```python
from build123d import *
from OCP.BRepFilletAPI import BRepFilletAPI_MakeChamfer

# Parameters (mm, degrees)
SKETCH_1_W               = 87
SKETCH_1_H               = 48
EXTRUDE_1_DEPTH          = 12
SKETCH_3_W               = 75
SKETCH_3_H               = 30
CUT_EXTRUDE_1_DEPTH      = 3
SKETCH_4_R               = 6
CUT_EXTRUDE_2_DEPTH      = 52.110175112
SKETCH_5_W               = 87
SKETCH_5_H               = 9
EXTRUDE_2_DEPTH          = 21
SKETCH_7_R               = 19.5
EXTRUDE_3_DEPTH          = 24
SKETCH_8_R               = 9
CUT_EXTRUDE_3_DEPTH      = 17
EXTRUDE_4_DEPTH          = 4.5
CUT_EXTRUDE_4_REACH      = 98.444
CUT_EXTRUDE_4_END_RADIUS = 9
SKETCH_13_R              = 3
CHAMFER_6_SIZE           = 1
CHAMFER_6_SIZE2          = 0.14060595
CHAMFER_6_SIZE2_2        = 0.017455065


with BuildPart() as part:
    # Sketch 1 → Extrude 1 (new body)
    with BuildSketch(Plane.XY):
        Rectangle(SKETCH_1_W, SKETCH_1_H)
    extrude(amount=-EXTRUDE_1_DEPTH)

    # Sketch 3 → Cut-Extrude 1 (cut)
    with BuildSketch(Plane(origin=(0, 0, -12), x_dir=(-1, 0, 0), z_dir=(0, 0, -1))):
        Rectangle(SKETCH_3_W, SKETCH_3_H)
    extrude(amount=-CUT_EXTRUDE_1_DEPTH, mode=Mode.SUBTRACT)

    # Sketch 4 → Cut-Extrude 2 (cut, through all)
    with BuildSketch(Plane.XY):
        with Locations((24, 0)):
            Circle(SKETCH_4_R)
        with Locations((-24, 0)):
            Circle(SKETCH_4_R)
    extrude(amount=-CUT_EXTRUDE_2_DEPTH, mode=Mode.SUBTRACT)

    # Sketch 5 → Extrude 2 (add)
    with BuildSketch(Plane(origin=(0, 0, -12), x_dir=(-1, 0, 0), z_dir=(0, 0, -1))):
        with Locations((0, -19.5)):
            Rectangle(SKETCH_5_W, SKETCH_5_H)
    extrude(amount=EXTRUDE_2_DEPTH)



with BuildPart() as body_2:
    # Sketch 7 → Extrude 3 (new, symmetric)
    with BuildSketch(Plane.XY.offset(-6)):
        with Locations((0, -75)):
            Circle(SKETCH_7_R)
    extrude(amount=EXTRUDE_3_DEPTH, both=True)

    # Sketch 8 → Cut-Extrude 3 (cut, symmetric)
    with BuildSketch(Plane.XY.offset(-6)):
        with Locations((0, -75)):
            Circle(SKETCH_8_R)
    extrude(amount=CUT_EXTRUDE_3_DEPTH, both=True, mode=Mode.SUBTRACT)

    # Sketch 10 → Cut-Revolve 1 (revolve, cut)
    with BuildSketch(Plane(origin=(0, -75, 0), x_dir=(1, 0, 0), z_dir=(0, 1, 0))):
        Polygon((0, -18), (0, -11), (9, -11), (10, -18), align=None)
    cut_revolve_1 = revolve(axis=Axis((0, -75, 18), (0, 0, -1)), mode=Mode.SUBTRACT)

    # Mirror 1: Cut-Revolve 1 across plane
    add(cut_revolve_1.mirror(Plane.XY.offset(-6)), mode=Mode.SUBTRACT)


with BuildPart() as part_1:
    add(part.part)

    add(body_2.part)  # Extrude 4 merges body 2
    # Sketch 12 → Extrude 4 (add, symmetric)
    with BuildSketch(Plane.XY.offset(-6)):
        with BuildLine():
            Line((-29.942238006, -27.63856044), (-15.687432014, -60.934386997))
            ThreePointArc((-15.687432014, -60.934386997), (-15.461093284, -62.422417649), (-15.985936875, -63.83309254))
            ThreePointArc((-15.985936875, -63.83309254), (0, -55.5), (15.985936875, -63.83309254))
            ThreePointArc((15.985936875, -63.83309254), (15.461093284, -62.422417649), (15.687432014, -60.934386997))
            Line((15.687432014, -60.934386997), (29.942238006, -27.63856044))
            ThreePointArc((29.942238006, -27.63856044), (32.154108719, -24.99157523), (35.457997537, -24))
            Line((35.457997537, -24), (-35.457997537, -24))
            ThreePointArc((-35.457997537, -24), (-32.154108719, -24.99157523), (-29.942238006, -27.63856044))
        make_face()
    extrude(amount=EXTRUDE_4_DEPTH, both=True)

    # Cut-Extrude 4: up to this cylinder (the profile starts outside it)
    cut_extrude_4_end = Plane(origin=(0, -75, 6), z_dir=(0, 0, 1)) * Cylinder(CUT_EXTRUDE_4_END_RADIUS, 215.888, mode=Mode.PRIVATE)
    # Sketch 13 → Cut-Extrude 4 (cut, up to the surface)
    with BuildSketch(Plane(origin=(0, -55.5, 0), x_dir=(1, 0, 0), z_dir=(0, 1, 0)), mode=Mode.PRIVATE) as cut_extrude_4_sk1:
        with Locations(Location((0, -6, 0), (0, 0, 270))):
            Circle(SKETCH_13_R)
    cut_extrude_4_tool1 = extrude(cut_extrude_4_sk1.sketch, amount=-CUT_EXTRUDE_4_REACH, mode=Mode.PRIVATE) - cut_extrude_4_end
    add(cut_extrude_4_tool1.solids().sort_by_distance((0, -55.5, 6))[0], mode=Mode.SUBTRACT)

    # Sketch 14 → Cut-Revolve 2 (revolve, cut)
    with BuildSketch(Plane.XY.offset(6), mode=Mode.PRIVATE) as cut_revolve_2_sk:
        Polygon((0, -55.5), (0, -57.5), (3, -57.5), (4.5, -55.5), align=None)
    revolve(cut_revolve_2_sk.sketch.rotate(Axis((0, -55.5, 6), (0, -1, 0)), 90), axis=Axis((0, -55.5, 6), (0, -1, 0)), mode=Mode.SUBTRACT)

    # Chamfer 6: one chamfer whose edges measure the first distance from different faces: ONE call of the kernel's chamfer builder (chamfer() names one face for all edges)
    chamfer_6_edges_1 = [part_1.edges().sort_by_distance(p)[0] for p in [
        (-9, -75, 11),
    ]]
    chamfer_6_side_1 = [part_1.faces().sort_by_distance(p)[0] for p in [
        (-9.5, -75, 14.5),
    ]]
    chamfer_6_edges_2 = [part_1.edges().sort_by_distance(p)[0] for p in [
        (-19.5, -75, -30),
    ]]
    chamfer_6_side_2 = [part_1.faces().sort_by_distance(p)[0] for p in [
        (-18.948456711, -75, -30),
    ]]
    chamfer_6_edges_3 = [part_1.edges().sort_by_distance(p)[0] for p in [
        (-19.5, -75, 18),
    ]]
    chamfer_6_side_3 = [part_1.faces().sort_by_distance(p)[0] for p in [
        (-19.5, -75, -6),
    ]]
    chamfer_6_edges_4 = [part_1.edges().sort_by_distance(p)[0] for p in [
        (-9, -75, -23),
    ]]
    chamfer_6_side_4 = [part_1.faces().sort_by_distance(p)[0] for p in [
        (-9, -75, -6),
    ]]
    chamfer_6 = BRepFilletAPI_MakeChamfer(part_1.part.solid().wrapped)
    for e in chamfer_6_edges_1:
        chamfer_6.Add(CHAMFER_6_SIZE, CHAMFER_6_SIZE2, e.wrapped, chamfer_6_side_1[0].wrapped)  # the first distance lies on this face
    for e in chamfer_6_edges_2:
        chamfer_6.Add(CHAMFER_6_SIZE, CHAMFER_6_SIZE2_2, e.wrapped, chamfer_6_side_2[0].wrapped)  # the first distance lies on this face
    for e in chamfer_6_edges_3:
        chamfer_6.Add(CHAMFER_6_SIZE, CHAMFER_6_SIZE2_2, e.wrapped, chamfer_6_side_3[0].wrapped)  # the first distance lies on this face
    for e in chamfer_6_edges_4:
        chamfer_6.Add(CHAMFER_6_SIZE, CHAMFER_6_SIZE2, e.wrapped, chamfer_6_side_4[0].wrapped)  # the first distance lies on this face
    add(Compound.cast(chamfer_6.Shape()), mode=Mode.REPLACE)


solid = part_1.part
```
Can you work these out from the model? Positions are in its coordinate system, mm. A direction names the side the tool comes from. Coordinates: 2 decimals unless noted, no trailing zeros. Loops run counter-clockwise (first coordinate to the right, second up) from the corner with the lowest first, then second, coordinate; pieces in that order, holes last.
Item 1: Suppose I cut it at C-C (x = -24). Please give me the cut outline in (y, z).
Answers below:
outline: (-41.52, -10.5) - (-24, -10.5) - (-24, -33) - (-15, -33) - (-15, -9) - (-6, -9) - (-6, 0) - (-24, 0) - (-24, -1.5) - (-41.52, -1.5) - close; (6, -9) - (15, -9) - (15, -12) - (24, -12) - (24, 0) - (6, 0) - close
Item 2: Which directions (+Z, -Z, +X, -X, +Y, -Y) give clear straight access to the entire face, cutting with the end or side of a thin tool? Please do faces 5 (the face through (37.5, 0, -11)), 6 (the face through (-1, 18, -12)), 7 (the face through (-4.227, -94.036, -6.162)), 8 (the face through (-1, 0, 0)).
Answers below:
face 5: -Z
face 6: -Z, +X, -X, +Y
face 7: none
face 8: +Z, +X, -X, +Y
Item 3: If we mould it in two halves opening along Y, with no side actions, what happens to faces 1 (the face through (-1.15, -61.94, 8.77)), 2 (the face through (1, 15, -11)), 3 (the face through (0, -39, -1.5)), 4 (the face through (-1, 24, -6))? For each: released by +Y, released by -Y, zero draft, split by the parting line, or undercut.
Answers below:
face 1: zero draft
face 2: undercut
face 3: undercut
face 4: released by +Y
Item 4: I'm going to push flat-ended pins straight in: pin 1 (3 mm diameter, centred on y = -79.5, z = -20.5, fed in from +X); pin 2 (12 mm diameter, centred on x = -1.5, y = -36, fed in from +Z); pin 3 (12 mm diameter, centred on y = -71, z = -9, fed in from +X); pin 4 (12 mm diameter, centred on y = 7, z = 3.5, fed in from +X). Where does each tip first touch, or does it pass through?
Answers below:
pin 1: stops at x = 19.27
pin 2: stops at z = -1.5
pin 3: stops at x = 19.5
pin 4: stops at x = 43.5
Item 5: Please list where these lines run through material, in increasing order: L1, parallel to Z at x = 0, y = -60.5; L2, parallel to Y at x = -5.5, z = -15; L3, parallel to Y at x = 20.5, z = -27.5.
Answers below:
L1: z = -30 to 3, 9 to 18
L2: y = -93.71 to -82.12, -67.88 to -56.29, -24 to -15
L3: y = -24 to -15
Item 6: Suppose I cut it at B-B (x = 26.5). Please give me the cut outline in (y, z).
Answers below:
outline: (-35.68, -10.5) - (-24, -10.5) - (-24, -33) - (-15, -33) - (-15, -9) - (-5.45, -9) - (-5.45, 0) - (-24, 0) - (-24, -1.5) - (-35.68, -1.5) - close; (5.45, -9) - (15, -9) - (15, -12) - (24, -12) - (24, 0) - (5.45, 0) - close
Item 7: Suppose I cut it at D-D (z = 6). Please give me the cut outline in (x, y), then the cut area to 4 significant figures.
Answers below:
outline: (-4.16, -55.95) arc R19.5 ccw (long way) to (4.16, -55.95) - (3, -57.5) - (3, -66.51) arc R9 cw (long way) to (-3, -66.51) - (-3, -57.5) - close
area: 874.5 mm2
Item 8: Suppose I cut it at A-A (y = 0). Please give me the cut outline in (x, z).
Answers below:
outline: (-43.5, -12) - (-37.5, -12) - (-37.5, -9) - (-30, -9) - (-30, 0) - (-43.5, 0) - close; (-18, -9) - (18, -9) - (18, 0) - (-18, 0) - close; (30, -9) - (37.5, -9) - (37.5, -12) - (43.5, -12) - (43.5, 0) - (30, 0) - close
